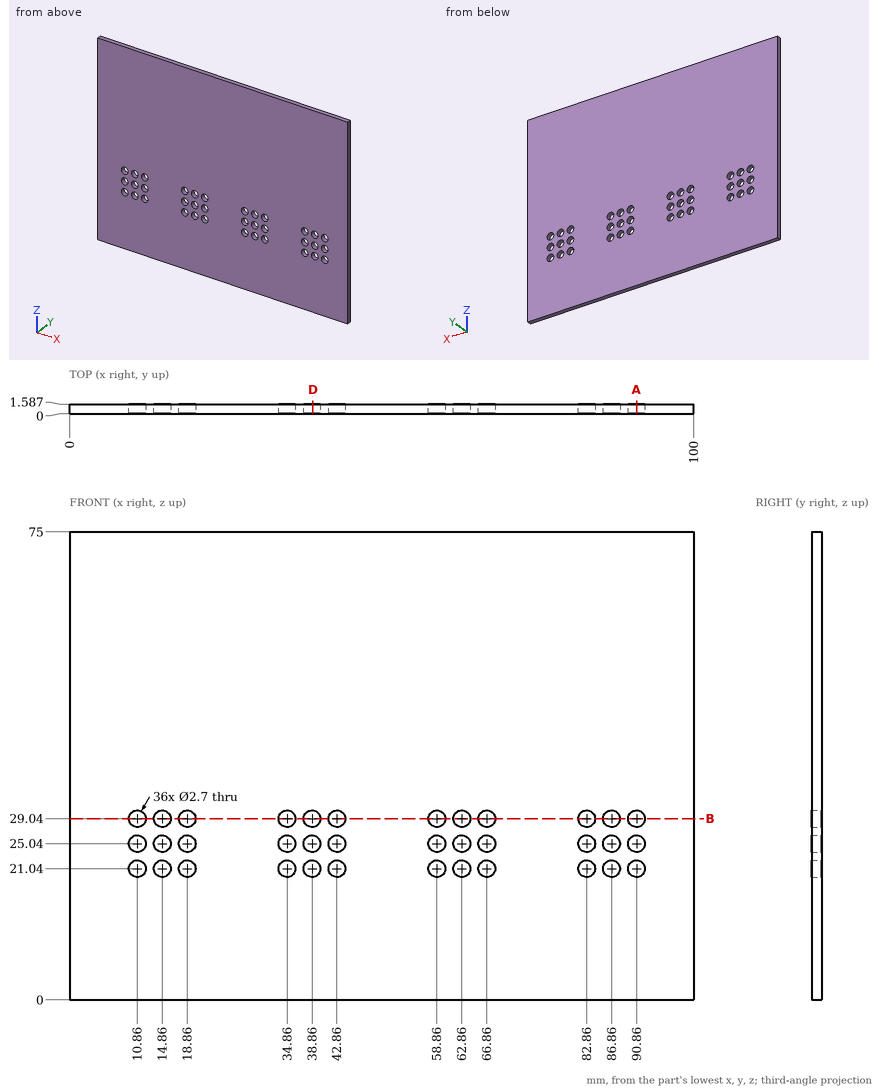
Can you work these out from the drawing? Everything is in mm from the part's minimum corner. Round coordinates to 2 decimals unless told otherwise and drop trailing zeros. Loops run counter-clockwise (first coordinate to the right, second up) from the corner with the lowest first, then second, coordinate; pieces in that order, holes last. Notation, with made-up numbers: (28.25, -30.75) - (54.25, -30.75) arc R18 cw to (54.25, -20.75) - close; hole circle Ø11 at (2, 72). An arc over 180 degrees is marked (long way). Answer as CSV lines item,"result".
1. I want a section at D-D on x = 39. List the corners of the cut face in (y, z) for me.
Filled in:
outline,"(0, 0) - (1.59, 0) - (1.59, 19.7) - (0, 19.7) - close; (0, 22.38) - (1.59, 22.38) - (1.59, 23.7) - (0, 23.7) - close; (0, 26.38) - (1.59, 26.38) - (1.59, 27.7) - (0, 27.7) - close; (0, 30.38) - (1.59, 30.38) - (1.59, 75) - (0, 75) - close"
2. I want a section at A-A on x = 90.86. List the corners of the cut face in (y, z) for me.
Filled in:
outline,"(0, 0) - (1.59, 0) - (1.59, 19.69) - (0, 19.69) - close; (0, 22.39) - (1.59, 22.39) - (1.59, 23.69) - (0, 23.69) - close; (0, 26.39) - (1.59, 26.39) - (1.59, 27.69) - (0, 27.69) - close; (0, 30.39) - (1.59, 30.39) - (1.59, 75) - (0, 75) - close"
3. I want a section at B-B on z = 29.04. Count the separate pieces of the cut face and the enclosed holes in it, then the cut area to 3 significant figures.
Filled in:
separate pieces,"13"
enclosed holes,"0"
area,"107 mm^2"
4. Please list where these lines run through material, in increasing order: line 1 along Z through (x, y) = (42.86, 1.2); line 2 along Z through (x, y) = (90, 0.1). Write a range as [from, to].
Filled in:
line 1,"z = [0, 19.69], [22.39, 23.69], [26.39, 27.69], [30.39, 75]"
line 2,"z = [0, 20], [22.08, 24], [26.08, 28], [30.08, 75]"
5. For pin 1 Ø2 at (x, z) = (90.86, 29.04) entering from -Y, with a flat end and sliding along its axis, tell me the tip position at first contact or that it passes through.
Filled in:
pin 1,"passes through"
